Geometry check sheet. Reference: drawing and pictorial views, mm from the part's lowest x, y, z. A direction names the side the tool comes from. Give positions to 0.01 mm unless a question says otherwise; leave off trailing zeros. Order: outer loops, then holes, each group sorted by start corner. A loop starts at its lowest first (then second) coordinate and runs counter-clockwise, first axis right, second up.
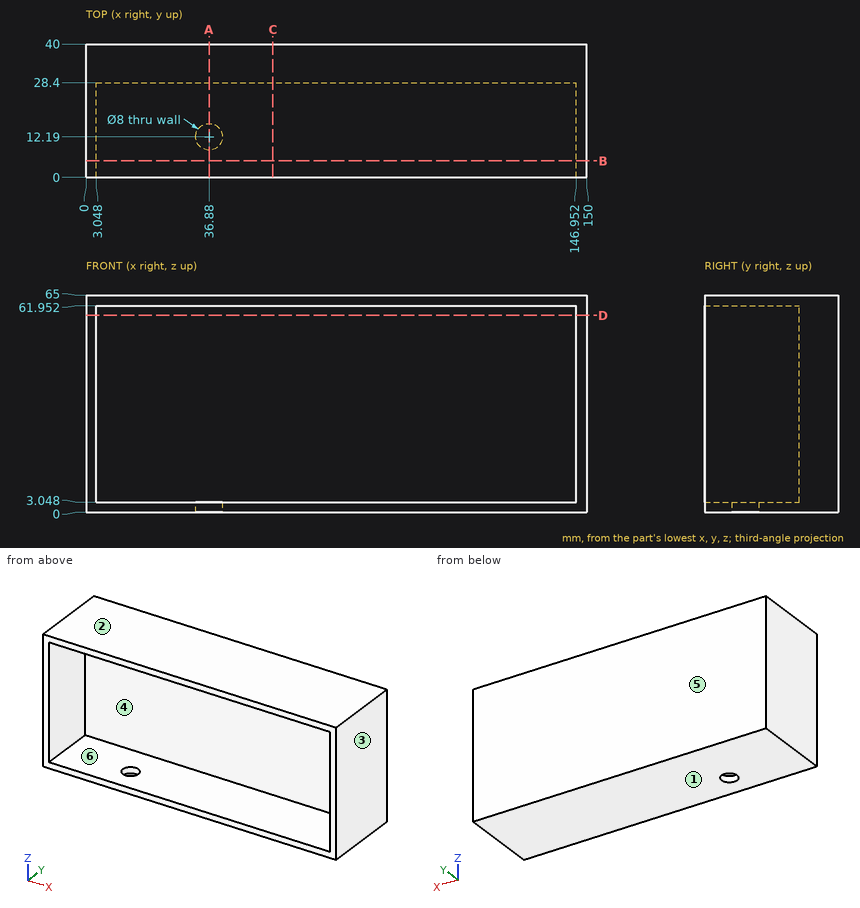
(1) Cross-section at D-D on z = 59. Enter the section's corners in (x, y).
Response values:
outline: (0, 0) - (3.05, 0) - (3.05, 28.4) - (146.95, 28.4) - (146.95, 0) - (150, 0) - (150, 40) - (0, 40) - close
(2) Cross-section at B-B on y = 5. Enter the section's corners in (x, z), then the cut area to 3 significant figures.
Response values:
outline: (0, 0) - (150, 0) - (150, 65) - (0, 65) - close; hole (3.05, 3.05) - (146.95, 3.05) - (146.95, 61.95) - (3.05, 61.95) - close
area: 1,270 mm2
(3) Cross-section at C-C on x = 56. Enter the section's corners in (y, z), then the cut area to 3 significant figures.
Response values:
outline: (0, 0) - (40, 0) - (40, 65) - (0, 65) - (0, 61.95) - (28.4, 61.95) - (28.4, 3.05) - (0, 3.05) - close
area: 927 mm2
(4) Cross-section at A-A on x = 36.88. Enter the section's corners in (y, z), then the cut area to 3 significant figures.
Response values:
outline: (0, 0) - (8.19, 0) - (8.19, 3.05) - (0, 3.05) - close; (0, 61.95) - (28.4, 61.95) - (28.4, 3.05) - (16.19, 3.05) - (16.19, 0) - (40, 0) - (40, 65) - (0, 65) - close
area: 903 mm2
(5) Release check for a two-part mould opening along Z. For the marked faces 1, 2, 3 and 4 record: released by +Z, released by -Z, zero draft, split by the parting line, or undercut.
Response values:
face 1: released by -Z
face 2: released by +Z
face 3: zero draft
face 4: undercut
(6) Set-up check for the marked faces 5 and 6: record each of +Z, -Z, +X, -X, +Y, -Y from which the full face is reachable in a straight line by a thin tool's end or side.
Response values:
face 5: +Z, -Z, +X, -X, +Y
face 6: -Y
(7) Material ranges on L1, parallel to Z at x = 75.5, y = 22; L2, parallel to X at y = 19.5, z = 19; L3, parallel to Y at x = 36.88, z = 1.25, recorded low to high.
Response values:
L1: z = 0 to 3.05, 61.95 to 65
L2: x = 0 to 3.05, 146.95 to 150
L3: y = 0 to 8.19, 16.19 to 40
